Check sheet for the drawn part. Datum: minimum x, y, z corner. Units: mm. A direction names the side the tool comes from. Coordinates: 2 decimals unless noted, no trailing zeros. Order: outer loops, then holes, each group sorted by start corner. A loop starts at its lowest first (then second) coordinate and runs counter-clockwise, first axis right, second up.
Q1. Cross-section at C-C, the plane z = 4.65. Record the boundary of the cut face in (x, y).
Q2. Cross-section at B-B, the plane x = 2.5. Record the boundary of the cut face in (y, z).
Q3. Depth check by flat-ended pin: P1, Ø2.5, axis at x = 2.5, y = 22, coming from the -Z side (3 decimals). Enter the tip coordinate at first touch or a pass-through.
Q4. Cross-section at D-D, the plane y = 9. Record the boundary of the cut face in (x, z).
Q5. Thickness scan on line 1 (Y direction, x = 2.5, z = 1.5); line 2 (X direction, y = 17, z = 2.15); line 3 (X direction, y = 10, z = 2). Record the ranges inside material, lowest first.
Q6. Set-up check for the marked faces 1 and 2: record each of +Z, -Z, +X, -X, +Y, -Y from which the full face is reachable in a straight line by a thin tool's end or side.
Q7. Draft check along X on the marked faces 3, 4 and 5. Enter one of: pulls with the +X half, pulls with the -X half, needs draft (parallel to the pull), parting line crosses it, or undercut.
Q8. Cross-section at A-A, the plane z = 0.75. Record the boundary of the cut face in (x, y), and give its area (3 significant figures).
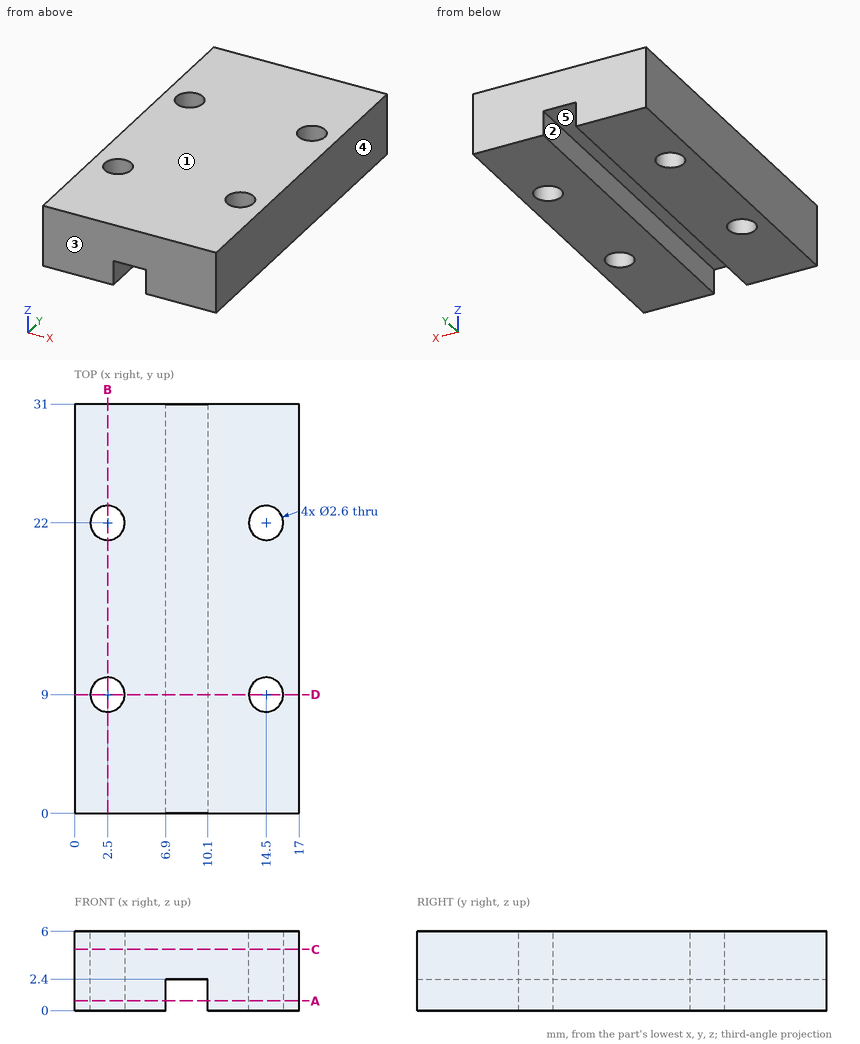
Check values:
1. outline: (0, 0) - (17, 0) - (17, 31) - (0, 31) - close; hole circle Ø2.6 at (2.5, 9); hole circle Ø2.6 at (2.5, 22); hole circle Ø2.6 at (14.5, 9); hole circle Ø2.6 at (14.5, 22)
2. outline: (0, 0) - (7.7, 0) - (7.7, 6) - (0, 6) - close; (10.3, 0) - (20.7, 0) - (20.7, 6) - (10.3, 6) - close; (23.3, 0) - (31, 0) - (31, 6) - (23.3, 6) - close
3. P1: passes through
4. outline: (0, 0) - (1.2, 0) - (1.2, 6) - (0, 6) - close; (3.8, 0) - (6.9, 0) - (6.9, 2.4) - (10.1, 2.4) - (10.1, 0) - (13.2, 0) - (13.2, 6) - (3.8, 6) - close; (15.8, 0) - (17, 0) - (17, 6) - (15.8, 6) - close
5. line 1: y = 0 to 7.7, 10.3 to 20.7, 23.3 to 31
5. line 2: x = 0 to 6.9, 10.1 to 17
5. line 3: x = 0 to 1.67, 3.33 to 6.9, 10.1 to 13.67, 15.33 to 17
6. face 1: +Z, +X, -X, +Y, -Y
6. face 2: -Z, +Y, -Y
7. face 3: needs draft
7. face 4: pulls with the +X half
7. face 5: undercut
8. outline: (0, 0) - (6.9, 0) - (6.9, 31) - (0, 31) - close; (10.1, 0) - (17, 0) - (17, 31) - (10.1, 31) - close; hole circle Ø2.6 at (2.5, 9); hole circle Ø2.6 at (2.5, 22); hole circle Ø2.6 at (14.5, 9); hole circle Ø2.6 at (14.5, 22)
8. area: 407 mm2
